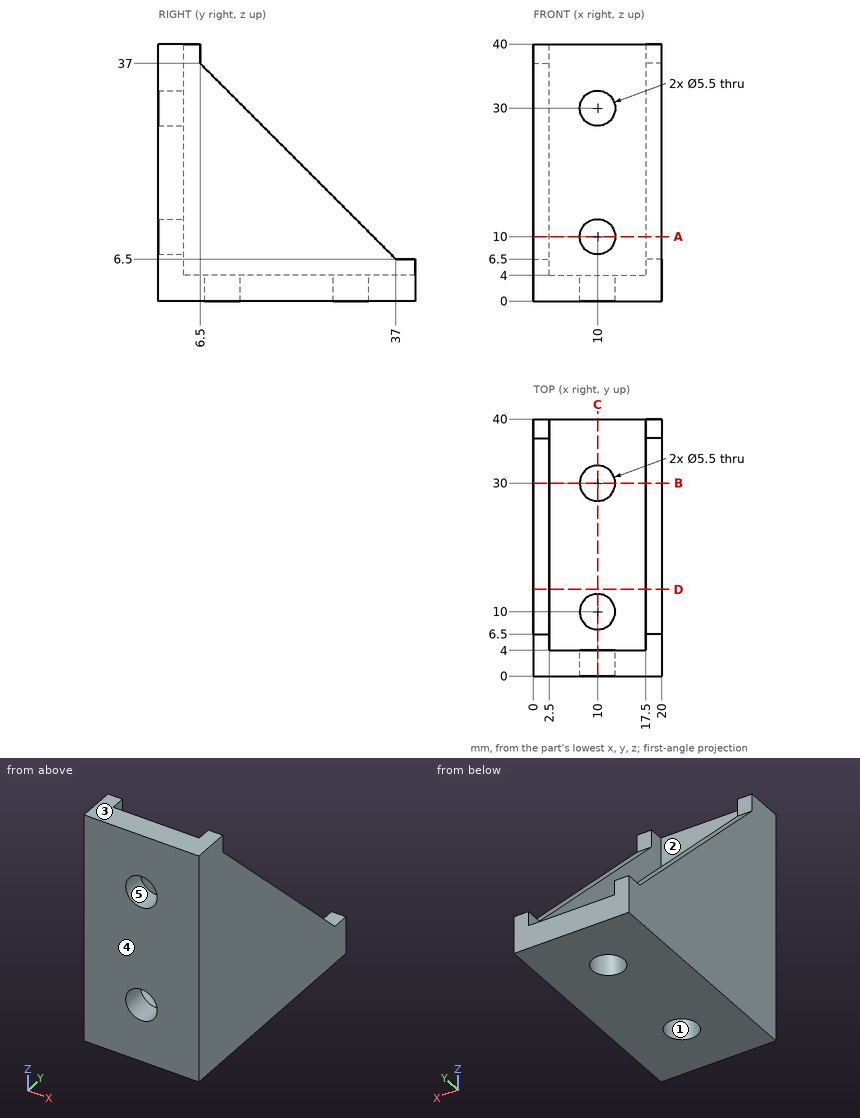
Check sheet for the drawn part. Datum: minimum x, y, z corner. Units: mm. A direction names the side the tool comes from. Round coordinates to 2 decimals unless told otherwise and drop trailing zeros. Order: outer loops, then holes, each group sorted by start corner. A loop starts at its lowest first (then second) coordinate and runs counter-clockwise, first axis right, second up.
1) Section check B-B (y = 30). Record the boundary of the cut face in (x, z), and give its area (4 significant figures).
2) Scan lines: line 1 (Z direction, x = 10, y = 1.55); line 2 (X direction, y = 30, z = 7). Record each from-to range of solid material in increasing order.
3) Section check A-A (z = 10). Record the boundary of the cut face in (x, y).
4) Go/stop test with flat-tipped pins: pin 1 Ø1.2 at (x, y) = (1, 38.5) entering from +Z; pin 2 Ø4.5 at (x, y) = (10, 10) entering from -Z; pin 3 Ø2 at (x, z) = (1, 39) entering from +Y; pin 4 Ø8 at (x, y) = (17, 34) entering from +Z. Record where each tip stops, or that it passes through.
5) Tool access check on the marked faces 1 and 2. Record the directions out of +Z, -Z, +X, -X, +Y, -Y that give a thin tool (end or side, any length) a straight path to the whole face; none if there is none.
6) Mould release check, pull along Z, two halves, no side actions. Record for the marked faces 3, 4 and 5: +Z half, -Z half, draft (parallel to the pull), parting line (faces both ways), or undercut.
7) Section check C-C (x = 10). Record the boundary of the cut face in (y, z).
8) Section check D-D (y = 13.5). Record the boundary of the cut face in (x, z), and give its area (3 significant figures).
Result:
1. outline: (0, 0) - (7.25, 0) - (7.25, 4) - (2.5, 4) - (2.5, 13.5) - (0, 13.5) - close; (12.75, 0) - (20, 0) - (20, 13.5) - (17.5, 13.5) - (17.5, 4) - (12.75, 4) - close
1. area: 105.5 mm2
2. line 1: z = 0 to 7.25, 12.75 to 27.25, 32.75 to 40
2. line 2: x = 0 to 2.5, 17.5 to 20
3. outline: (0, 0) - (7.25, 0) - (7.25, 4) - (2.5, 4) - (2.5, 33.5) - (0, 33.5) - close; (12.75, 0) - (20, 0) - (20, 33.5) - (17.5, 33.5) - (17.5, 4) - (12.75, 4) - close
4. pin 1: stops at z = 6.5
4. pin 2: passes through
4. pin 3: stops at y = 6.5
4. pin 4: stops at z = 13.47
5. face 1: +Z, -Z
5. face 2: +Z, +Y
6. face 3: +Z half
6. face 4: draft
6. face 5: undercut
7. outline: (0, 0) - (7.25, 0) - (7.25, 4) - (4, 4) - (4, 7.25) - (0, 7.25) - close; (0, 12.75) - (4, 12.75) - (4, 27.25) - (0, 27.25) - close; (0, 32.75) - (4, 32.75) - (4, 40) - (0, 40) - close; (12.75, 0) - (27.25, 0) - (27.25, 4) - (12.75, 4) - close; (32.75, 0) - (40, 0) - (40, 4) - (32.75, 4) - close
8. outline: (0, 0) - (20, 0) - (20, 30) - (17.5, 30) - (17.5, 4) - (2.5, 4) - (2.5, 30) - (0, 30) - close
8. area: 210 mm2
